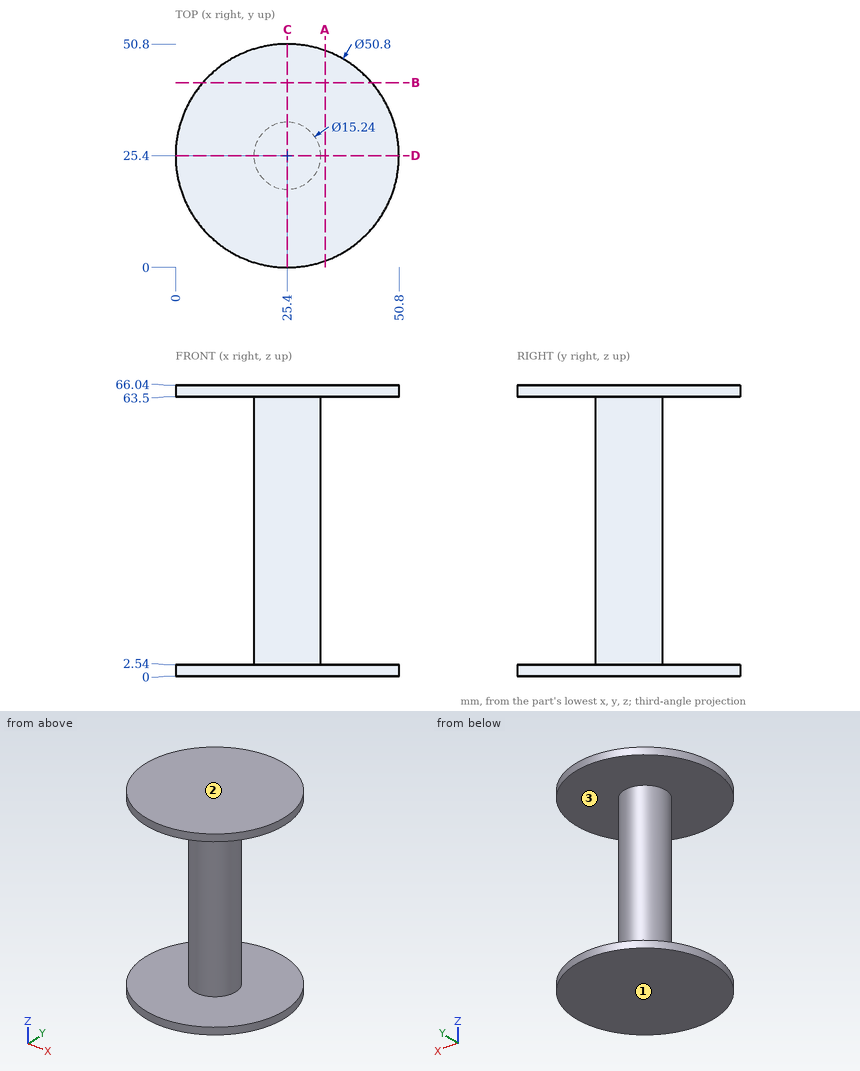
The drawing under review shows one solid part. Ordinate dimensions are in mm from its lowest x, y, z. Round coordinates to 2 decimals unless told otherwise and drop trailing zeros. Order: outer loops, then holes, each group sorted by start corner. A loop starts at its lowest first (then second) coordinate and runs counter-clockwise, first axis right, second up. Notation, with made-up numbers: (37, -16) -> (82, -16) arc R27 ccw to (82, 22) -> close; hole circle Ø1 at (68, -35.75). An arc over 180 degrees is marked (long way). Use a Markdown table: item, result.
Item 1: Take a section at B-B (y = 42). State the section outline as (x, z) points, plus the area to 3 significant figures.
Resolved:
| item | result |
|---|---|
| outline | (6.18, 0) -> (44.62, 0) -> (44.62, 2.54) -> (6.18, 2.54) -> close; (6.18, 63.5) -> (44.62, 63.5) -> (44.62, 66.04) -> (6.18, 66.04) -> close |
| area | 195 mm² |
Item 2: Take a section at C-C (x = 25.4). State the section outline as (y, z) points.
Resolved:
| item | result |
|---|---|
| outline | (0, 0) -> (50.8, 0) -> (50.8, 2.54) -> (33.02, 2.54) -> (33.02, 63.5) -> (50.8, 63.5) -> (50.8, 66.04) -> (0, 66.04) -> (0, 63.5) -> (17.78, 63.5) -> (17.78, 2.54) -> (0, 2.54) -> close |
Item 3: For pin 1 (4 mm diameter, centred on y = 25, z = 27.5, fed in from +X); pin 2 (12 mm diameter, centred on x = 29, z = 58, fed in from -Y); pin 3 (6 mm diameter, centred on x = 19, z = 27, fed in from -Y), all flat-tipped, find the tip position at first contact; note any pin that passes through.
Resolved:
| item | result |
|---|---|
| pin 1 | stops at x = 33.02 |
| pin 2 | stops at y = 0.03 |
| pin 3 | stops at y = 18.58 |
Item 4: Take a section at A-A (x = 34). State the section outline as (y, z) points.
Resolved:
| item | result |
|---|---|
| outline | (1.5, 0) -> (49.3, 0) -> (49.3, 2.54) -> (1.5, 2.54) -> close; (1.5, 63.5) -> (49.3, 63.5) -> (49.3, 66.04) -> (1.5, 66.04) -> close |
Item 5: For line 1 along Z through (x, y) = (14.5, 22); line 2 along X through (y, z) = (25, 17); line 3 along X through (y, z) = (20, 36.5), list the stretches that pass through material, from the lowest coordinate up. Write a range as [from, to].
Resolved:
| item | result |
|---|---|
| line 1 | z = [0, 2.54], [63.5, 66.04] |
| line 2 | x = [17.79, 33.01] |
| line 3 | x = [20.02, 30.78] |
Item 6: Draft analysis for pull direction Z (two halves, no side actions). For the marked faces 1, 2 and 3, state which applies: +Z half, -Z half, draft (parallel to the pull), parting line (faces both ways), or undercut.
Resolved:
| item | result |
|---|---|
| face 1 | -Z half |
| face 2 | +Z half |
| face 3 | undercut |
